Check sheet for the modelled part. Datum: model origin and axes. Units: mm. A direction names the side the tool comes from. Coordinates: 2 decimals unless noted, no trailing zeros. Loops run counter-clockwise (first coordinate to the right, second up) from the corner with the lowest first, then second, coordinate; pieces in that order, holes last. Notation, with made-up numbers: (85.5, -16.75) - (136.5, -16.75) arc R27 cw to (136.5, -0.75) - close; hole circle Ø1 at (27.5, 83). An arc over 180 degrees is marked (long way). Use a Markdown table: item, result. Add a question column.
1) Sectioned sample at A-A, the plane x = -76. Enter the section's corners in (y, z), then the cut area to 3 significant figures.
2) Sectioned sample at D-D, the plane x = 127. Enter the section's corners in (y, z), then the cut area to 3 significant figures.
3) Go/stop test with flat-tipped pins: P1, Ø15, axis at x = 517.5, y = -40, coming from the +Z side; P2, Ø1.6, axis at x = -151, z = 32, coming from the +Y side; P3, Ø24, axis at x = -228, y = 0, coming from the +Z side. Record where each tip stops, or that it passes through.
4) Sectioned sample at C-C, the plane z = 21. Enter the section's corners in (x, y), then the cut area to 3 significant figures.
5) Sectioned sample at B-B, the plane y = 0. Enter the section's corners in (x, z).
6) Draft check along X on faces 1 (the flat face through (-535, 0, -1)), 2 (the cylindrical face through (-88, -9, -1)), 3 (the flat face through (7, 80, 15)), 4 (the flat face through (535, 0, -1)). Enter one of: pulls with the +X half, pulls with the -X half, needs draft (parallel to the pull), parting line crosses it, or undercut.
7) Thickness scan on line 1 (Y direction, x = 239, z = 20.5); line 2 (Y direction, x = 76, z = -1); line 3 (Z direction, x = 55, y = -67). Record the ranges inside material, lowest first.
8) Tool access check on faces 5 (the flat face through (7, 78, 16)), 6 (the flat face through (-7, 1, -2)). Record the directions out of +Z, -Z, +X, -X, +Y, -Y that give a thin tool (end or side, any length) a straight path to the whole face; none if there is none.
from build123d import *

# Parameters (mm, degrees)
SKETCH1_W                      = 1070
SKETCH1_H                      = 160
BASE_FLANGE1_DEPTH             = 2
EDGE_FLANGE1_STRIP_W           = 14
EDGE_FLANGE1_STRIP_H           = 2
EDGE_FLANGE1_STRIP_CUT_DEPTH   = 1070
EDGE_FLANGE1_STRIP_2_W         = 14
EDGE_FLANGE1_STRIP_2_H         = 2
EDGE_FLANGE1_STRIP_CUT_2_DEPTH = 1070
EDGE_FLANGE1_DEPTH             = 1070
EDGE_FLANGE1_BEND_DEPTH        = 1070
EDGE_FLANGE2_STRIP_W           = 14
EDGE_FLANGE2_STRIP_H           = 2
EDGE_FLANGE2_STRIP_CUT_DEPTH   = 1070
EDGE_FLANGE2_STRIP_2_W         = 14
EDGE_FLANGE2_STRIP_2_H         = 2
EDGE_FLANGE2_STRIP_CUT_2_DEPTH = 1070
EDGE_FLANGE2_DEPTH             = 1070
EDGE_FLANGE2_BEND_DEPTH        = 1070
SKETCH18_R                     = 6.5
CUT_EXTRUDE1_DEPTH             = 10
SKETCH19_R                     = 15
CUT_EXTRUDE2_DEPTH             = 542.953872576
LPATTERN1_COUNT                = 6
LPATTERN1_PITCH                = 152


# Sheet-metal steps are written as plain solids
with BuildPart() as part:
    # Sketch1 → Base-Flange1 (new body)
    with BuildSketch(Plane.XY):
        Rectangle(SKETCH1_W, SKETCH1_H)
    extrude(amount=-BASE_FLANGE1_DEPTH)

    # Edge-Flange1 strip (across the edge) → Edge-Flange1 strip cut (cut)
    with BuildSketch(Plane(origin=(535, 80, 0), x_dir=(0, -1, 0), z_dir=(-1, 0, 0))):
        with Locations((-2, -1)):
            Rectangle(EDGE_FLANGE1_STRIP_W, EDGE_FLANGE1_STRIP_H)
    extrude(amount=EDGE_FLANGE1_STRIP_CUT_DEPTH, mode=Mode.SUBTRACT)

    # Edge-Flange1 strip 2 (across the edge) → Edge-Flange1 strip cut 2 (cut)
    with BuildSketch(Plane(origin=(-535, -80, 0), x_dir=(0, 1, 0), z_dir=(1, 0, 0))):
        with Locations((-2, -1)):
            Rectangle(EDGE_FLANGE1_STRIP_2_W, EDGE_FLANGE1_STRIP_2_H)
    extrude(amount=EDGE_FLANGE1_STRIP_CUT_2_DEPTH, mode=Mode.SUBTRACT)

    # Edge-Flange1 section (across the edge) → Edge-Flange1 (add)
    with BuildSketch(Plane(origin=(535, 80, 0), x_dir=(0, -1, 0), z_dir=(-1, 0, 0))):
        with BuildLine():
            Line((0, 3), (0, 33))
            Line((0, 33), (2, 33))
            Line((2, 33), (2, 3))
            ThreePointArc((2, 3), (2.878679656, 0.878679656), (5, 0))
            Line((5, 0), (5, -2))
            ThreePointArc((5, -2), (1.464466094, -0.535533906), (0, 3))
        make_face()
    extrude(amount=EDGE_FLANGE1_DEPTH)

    # Edge-Flange1 section 2 (across the edge) → Edge-Flange1 bend (add)
    with BuildSketch(Plane(origin=(-535, -80, 0), x_dir=(0, 1, 0), z_dir=(1, 0, 0))):
        with BuildLine():
            Line((0, 3), (0, 33))
            Line((0, 33), (2, 33))
            Line((2, 33), (2, 3))
            ThreePointArc((2, 3), (2.878679656, 0.878679656), (5, 0))
            Line((5, 0), (5, -2))
            ThreePointArc((5, -2), (1.464466094, -0.535533906), (0, 3))
        make_face()
    extrude(amount=EDGE_FLANGE1_BEND_DEPTH)

    # Edge-Flange2 strip (across the edge) → Edge-Flange2 strip cut (cut)
    with BuildSketch(Plane(origin=(-535, -78, 33), x_dir=(0, 0, -1), z_dir=(1, 0, 0))):
        with Locations((-2, -1)):
            Rectangle(EDGE_FLANGE2_STRIP_W, EDGE_FLANGE2_STRIP_H)
    extrude(amount=EDGE_FLANGE2_STRIP_CUT_DEPTH, mode=Mode.SUBTRACT)

    # Edge-Flange2 strip 2 (across the edge) → Edge-Flange2 strip cut 2 (cut)
    with BuildSketch(Plane(origin=(535, 78, 33), x_dir=(0, 0, -1), z_dir=(-1, 0, 0))):
        with Locations((-2, -1)):
            Rectangle(EDGE_FLANGE2_STRIP_2_W, EDGE_FLANGE2_STRIP_2_H)
    extrude(amount=EDGE_FLANGE2_STRIP_CUT_2_DEPTH, mode=Mode.SUBTRACT)

    # Edge-Flange2 section (across the edge) → Edge-Flange2 (add)
    with BuildSketch(Plane(origin=(-535, -78, 33), x_dir=(0, 0, -1), z_dir=(1, 0, 0))):
        with BuildLine():
            Line((0, 3), (0, 13))
            Line((0, 13), (2, 13))
            Line((2, 13), (2, 3))
            ThreePointArc((2, 3), (2.878679656, 0.878679656), (5, 0))
            Line((5, 0), (5, -2))
            ThreePointArc((5, -2), (1.464466094, -0.535533906), (0, 3))
        make_face()
    extrude(amount=EDGE_FLANGE2_DEPTH)

    # Edge-Flange2 section 2 (across the edge) → Edge-Flange2 bend (add)
    with BuildSketch(Plane(origin=(535, 78, 33), x_dir=(0, 0, -1), z_dir=(-1, 0, 0))):
        with BuildLine():
            Line((0, 3), (0, 13))
            Line((0, 13), (2, 13))
            Line((2, 13), (2, 3))
            ThreePointArc((2, 3), (2.878679656, 0.878679656), (5, 0))
            Line((5, 0), (5, -2))
            ThreePointArc((5, -2), (1.464466094, -0.535533906), (0, 3))
        make_face()
    extrude(amount=EDGE_FLANGE2_BEND_DEPTH)

    # Sketch18 → Cut-Extrude1 (cut)
    with BuildSketch(Plane.XY):
        with Locations((-517.5, 40)):
            Circle(SKETCH18_R)
        with Locations((-517.5, -40)):
            Circle(SKETCH18_R)
        with Locations((517.5, -40)):
            Circle(SKETCH18_R)
        with Locations((517.5, 40)):
            Circle(SKETCH18_R)
    extrude(amount=-CUT_EXTRUDE1_DEPTH, mode=Mode.SUBTRACT)

    # Sketch19 → Cut-Extrude2 (cut, symmetric)
    with BuildSketch(Plane.XY):
        with Locations((380, 0)):
            Circle(SKETCH19_R)
    cut_extrude2 = extrude(amount=CUT_EXTRUDE2_DEPTH, both=True, mode=Mode.SUBTRACT)

    # LPattern1: Cut-Extrude2 ×6
    with Locations(*[(-i * LPATTERN1_PITCH, 0, 0) for i in range(1, LPATTERN1_COUNT)]):
        add(cut_extrude2, mode=Mode.SUBTRACT)


solid = part.part
Solved:
| question | item | result |
|---|---|---|
| 1 | outline | (-80, 3) arc R5 ccw to (-75, -2) - (-15, -2) - (-15, 0) - (-75, 0) arc R3 cw to (-78, 3) - (-78, 28) arc R3 cw to (-75, 31) - (-65, 31) - (-65, 33) - (-75, 33) arc R5 ccw to (-80, 28) - close; (15, -2) - (75, -2) arc R5 ccw to (80, 3) - (80, 28) arc R5 ccw to (75, 33) - (65, 33) - (65, 31) - (75, 31) arc R3 cw to (78, 28) - (78, 3) arc R3 cw to (75, 0) - (15, 0) - close |
| 1 | area | 430 mm2 |
| 2 | outline | (-80, 3) arc R5 ccw to (-75, -2) - (75, -2) arc R5 ccw to (80, 3) - (80, 28) arc R5 ccw to (75, 33) - (65, 33) - (65, 31) - (75, 31) arc R3 cw to (78, 28) - (78, 3) arc R3 cw to (75, 0) - (-75, 0) arc R3 cw to (-78, 3) - (-78, 28) arc R3 cw to (-75, 31) - (-65, 31) - (-65, 33) - (-75, 33) arc R5 ccw to (-80, 28) - close |
| 2 | area | 490 mm2 |
| 3 | P1 | stops at z = 0 |
| 3 | P2 | stops at y = 78.84 |
| 3 | P3 | passes through |
| 4 | outline | (-535, -80) - (535, -80) - (535, -78) - (-535, -78) - close; (-535, 78) - (535, 78) - (535, 80) - (-535, 80) - close |
| 4 | area | 4,280 mm2 |
| 5 | outline | (-535, -2) - (-395, -2) - (-395, 0) - (-535, 0) - close; (-365, -2) - (-243, -2) - (-243, 0) - (-365, 0) - close; (-213, -2) - (-91, -2) - (-91, 0) - (-213, 0) - close; (-61, -2) - (61, -2) - (61, 0) - (-61, 0) - close; (91, -2) - (213, -2) - (213, 0) - (91, 0) - close; (243, -2) - (365, -2) - (365, 0) - (243, 0) - close; (395, -2) - (535, -2) - (535, 0) - (395, 0) - close |
| 6 | face 1 | pulls with the -X half |
| 6 | face 2 | undercut |
| 6 | face 3 | needs draft |
| 6 | face 4 | pulls with the +X half |
| 7 | line 1 | y = -80 to -78, 78 to 80 |
| 7 | line 2 | y = -78 to -15, 15 to 78 |
| 7 | line 3 | z = -2 to 0, 31 to 33 |
| 8 | face 5 | +X, -X |
| 8 | face 6 | -Z, +X, -X, +Y, -Y |
